Autodesk Inventor part; units mm, degrees
ref_plane "YZ Plane" through (0, 0, 0) normal (1, 0, 0) x (0, 1, 0)
ref_plane "XZ Plane" through (0, 0, 0) normal (0, 1, 0) x (-1, 0, 0)
ref_plane "XY Plane" through (0, 0, 0) normal (0, 0, 1) x (1, 0, 0)
sketch "Sketch1" plane through (0, 0, 0) normal (0, 0, 1) x (1, 0, 0)
  line L0 (0, 0) -> (145.9, 0)
  line L1 (145.9, 0) -> (145.9, 75.9)
  line L2 (145.9, 75.9) -> (0, 75.9)
  line L3 (0, 75.9) -> (0, 0)
  dimension "d0" = 145.9
  dimension "d1" = 75.9
extrude "Extrusion1" add sketch "Sketch1" along normal blind 1
sketch "Sketch2" plane through (0, 0, 1) normal (0, 0, 1) x (1, 0, 0)
  line L0 (145.9, 75.9) -> (0, 75.9) construction
  line L1 (0, 75.9) -> (0, 0) construction
  line L2 (0, 0) -> (145.9, 0) construction
  line L3 (145.9, 0) -> (145.9, 75.9) construction
  line L4 (145.9, 75.9) -> (0, 75.9) construction
  line L5 (0, 75.9) -> (0, 0) construction
  line L6 (141.05, 4.85) -> (4.85, 4.85) construction
  line L7 (4.85, 4.85) -> (4.85, 71.05) construction
  line L8 (4.85, 71.05) -> (141.05, 71.05) construction
  line L9 (141.05, 71.05) -> (141.05, 4.85) construction
  dimension "d4" = 4.85
hole "Hole1" at (4.85, 71.05, 1) at (4.85, 4.85, 1) at (141.05, 4.85, 1) at (141.05, 71.05, 1) direction (0, 0, -1) diameter 3 end through all
sketch "Sketch3" plane through (0, 0, 0) normal (0, 0, -1) x (-1, 0, 0)
  circle A0 centre (-141.05, 4.85) radius 1.5 construction
  circle A1 centre (-4.85, 71.05) radius 1.5 construction
  circle A2 centre (-4.85, 4.85) radius 1.5 construction
  circle A3 centre (-141.05, 71.05) radius 1.5 construction
  line L0 (0, 0) -> (-145.9, 0) construction
  line L1 (0, 75.9) -> (0, 0) construction
  line L2 (-145.9, 75.9) -> (0, 75.9) construction
  line L3 (-145.9, 0) -> (-145.9, 75.9) construction
  line L4 (-68.15, 0) -> (-68.15, 75.9) construction
  line L5 (0, 9.45) -> (-68.15, 9.45) construction
  line L6 (0, 28.45) -> (-68.15, 28.45) construction
  line L7 (0, 47.45) -> (-68.15, 47.45) construction
  line L8 (0, 66.45) -> (-68.15, 66.45) construction
  circle A4 centre (-68.15, 9.45) radius 7.5
  circle A5 centre (-68.15, 28.45) radius 7.5
  circle A6 centre (-68.15, 47.45) radius 7.5
  circle A7 centre (-68.15, 66.45) radius 7.5
  dimension "d20" = 68.15
  dimension "d21" = 9.45
  dimension "d23" = 19
  dimension "d24" = 19
  dimension "d25" = 19
  dimension "d26" = 15
  dimension "d27" = 15
  dimension "d28" = 15
  dimension "d29" = 15
extrude "Extrusion2" cut sketch "Sketch3" against normal blind 0.001
properties part number "Polycarbonate Facia" material "Polycarbonate, Clear"
Design review of the part built by this model. Coordinates are the model's own, in mm. Give positions to 0.01 mm unless a question says otherwise; leave off trailing zeros. Use CSV: the item, a comma, the result in double quotes. Start each with the question number.
1. Add section A-A (y = 71.05). Count the separate pieces of the cut face and the enclosed holes in it, plus the area to 3 significant figures.
2. Wall thickness on L1, parallel to X at y = 71.05, z = 0.5; L2, parallel to Y at x = 141.05, z = 0.5; L3, parallel to X at y = 70.5, z = 0.4: over which ranges is each line inside the solid? List them lowest first.
3. Draft analysis for pull direction X (two halves, no side actions). For faces 1 (the flat face through (72, 38, 0)), 2 (the cylindrical face through (139.785, 4.044, 0.493)), state which applies: released by +X, released by -X, zero draft, split by the parting line, or undercut.
4. Insertion check: P1, Ø12, axis at x = 115.5, y = 36, coming from the -Z side. The pin has a flat end and moves straight along its axis. Give the tip position at first contact, or say it passes through.
Results found:
1,separate pieces,"3"
1,enclosed holes,"0"
1,area,"140 mm²"
2,L1,"x = 0 to 3.35, 6.35 to 139.55, 142.55 to 145.9"
2,L2,"y = 0 to 3.35, 6.35 to 69.55, 72.55 to 75.9"
2,L3,"x = 0 to 3.45, 6.25 to 139.65, 142.45 to 145.9"
3,face 1,"zero draft"
3,face 2,"undercut"
4,P1,"stops at z = 0"
